Design review of the part built by this model. Coordinates are the model's own, in mm. A direction names the side the tool comes from. Give positions to 0.01 mm unless a question says otherwise; leave off trailing zeros. Order: outer loops, then holes, each group sorted by start corner. A loop starts at its lowest first (then second) coordinate and runs counter-clockwise, first axis right, second up.
Autodesk Inventor part; units mm, degrees
ref_plane "YZ Plane" through (0, 0, 0) normal (1, 0, 0) x (0, 1, 0)
ref_plane "XZ Plane" through (0, 0, 0) normal (0, 1, 0) x (-1, 0, 0)
ref_plane "XY Plane" through (0, 0, 0) normal (0, 0, 1) x (1, 0, 0)
sketch "Sketch1" plane through (0, 0, 0) normal (0, 0, 1) x (1, 0, 0)
  line L0 (0, 0) -> (18, 0)
  line L1 (18, 0) -> (18, 18)
  line L2 (18, 18) -> (0, 18)
  line L3 (0, 18) -> (0, 0)
  dimension "d0" = 18
  dimension "d1" = 18
extrude "Extrusion1" add sketch "Sketch1" along normal blind 16
sketch "Sketch2" plane through (18, 0, 0) normal (1, 0, 0) x (0, 0, -1)
  line L0 (-16, 0) -> (-12, 0)
  line L1 (0, 0) -> (-16, 0)
  line L2 (-12, 0) -> (-12, 3)
  line L3 (-12, 3) -> (-4, 3)
  line L4 (-4, 3) -> (-4, 0)
  line L5 (-16, 0) -> (-16, 18)
  line L6 (-16, 18) -> (-12, 18)
  line L7 (0, 18) -> (-16, 18)
  line L8 (-12, 15) -> (-4, 15)
  line L9 (-4, 15) -> (-4, 18)
  line L10 (-12, 18) -> (-12, 15)
  dimension "d4" = 4
  dimension "d5" = 3
  dimension "d6" = 8
  dimension "d7" = 4
  dimension "d8" = 8
  dimension "d9" = 3
extrude "Extrusion2" cut sketch "Sketch2" against normal through all
sketch "Sketch3" plane through (18, 0, 0) normal (1, 0, 0) x (0, 0, -1)
  line L0 (-13, 12) -> (-3, 12)
  line L1 (-3, 12) -> (-3, 6)
  line L2 (-3, 6) -> (-13, 6)
  line L3 (-13, 6) -> (-13, 12)
  line L4 (0, 0) -> (0, 18)
  line L5 (-16, 0) -> (-16, 18)
  line L6 (-4, 15) -> (-12, 15)
  line L7 (-12, 3) -> (-4, 3)
  dimension "d12" = 3
  dimension "d13" = 3
  dimension "d14" = 3
  dimension "d15" = 3
extrude "Extrusion3" cut sketch "Sketch3" against normal through all
sketch "Sketch4" plane through (18, 15, 12) normal (0, 1, 0) x (1, 0, 0)
  circle A0 centre (-9, 4) radius 1.5
  line L0 (-18, 8) -> (0, 8)
  line L1 (-18, 0) -> (-18, 8)
  point P0 (-18, 12)
  dimension "d18" = 3
  dimension "d19" = 4
  dimension "d20" = 9
extrude "Extrusion4" cut sketch "Sketch4" against normal through all
equation "\"d7\" = d4"
equation "\"d8\" = d6"
equation "\"d9\" = d5"
equation "\"d13\" = d12"
equation "\"d15\" = d14"
properties part number "BeamConnectionPoint"
1. Take a section at B-B (x = 2.5). State the section outline as (y, z) points.
Recorded:
outline: (0, 0) - (18, 0) - (18, 4) - (15, 4) - (15, 12) - (18, 12) - (18, 16) - (0, 16) - (0, 12) - (3, 12) - (3, 4) - (0, 4) - close; hole (6, 3) - (12, 3) - (12, 13) - (6, 13) - close
2. Take a section at D-D (x = 9). State the section outline as (y, z) points.
Recorded:
outline: (0, 0) - (18, 0) - (18, 4) - (15, 4) - (15, 6.5) - (12, 6.5) - (12, 3) - (6, 3) - (6, 6.5) - (3, 6.5) - (3, 4) - (0, 4) - close; (0, 12) - (3, 12) - (3, 9.5) - (6, 9.5) - (6, 13) - (12, 13) - (12, 9.5) - (15, 9.5) - (15, 12) - (18, 12) - (18, 16) - (0, 16) - close
3. Take a section at C-C (y = 9.5). State the section outline as (x, z) points, then the cut area to 3 significant figures.
Recorded:
outline: (0, 0) - (18, 0) - (18, 3) - (0, 3) - close; (0, 13) - (18, 13) - (18, 16) - (0, 16) - close
area: 108 mm2
4. For line 1 along Y through (x, z) = (1.5, 8.5); line 2 along Z through (x, y) = (9, 4.15); line 3 along Y through (x, z) = (2.5, 12.75), list the stretches that pass through material, from the lowest coordinate up.
Recorded:
line 1: y = 3 to 6, 12 to 15
line 2: z = 0 to 6.5, 9.5 to 16
line 3: y = 0 to 6, 12 to 18
5. Take a section at A-A (z = 5). State the section outline as (x, y) points, then the cut area to 3 significant figures.
Recorded:
outline: (0, 3) - (18, 3) - (18, 6) - (0, 6) - close; (0, 12) - (18, 12) - (18, 15) - (0, 15) - close
area: 108 mm2
6. Draft analysis for pull direction Z (two halves, no side actions). For faces 6 (the face through (9, 9, 0)), 7 (the face through (9, 1, 12)), 8 (the face through (9, 17, 12)), 9 (the face through (9, 18, 14)), state which applies: pulls with the +Z half, pulls with the -Z half, needs draft (parallel to the pull), parting line crosses it, or undercut.
Recorded:
face 6: pulls with the -Z half
face 7: undercut
face 8: undercut
face 9: needs draft
7. Machinability: for faces 1 (the face through (9, 18, 2)), 2 (the face through (7, 6, 8)), 3 (the face through (18, 13, 8)), 4 (the face through (9, 2, 4)), 5 (the face through (9, 16, 4)), which of the approach directions +Z, -Z, +X, -X, +Y, -Y give a long, thin tool a straight path to every point of the face, cutting with its end or side? Answer none if there is none.
Recorded:
face 1: +Z, -Z, +X, -X, +Y
face 2: +X, -X
face 3: +Z, -Z, +X, +Y, -Y
face 4: +X, -X, -Y
face 5: +X, -X, +Y
